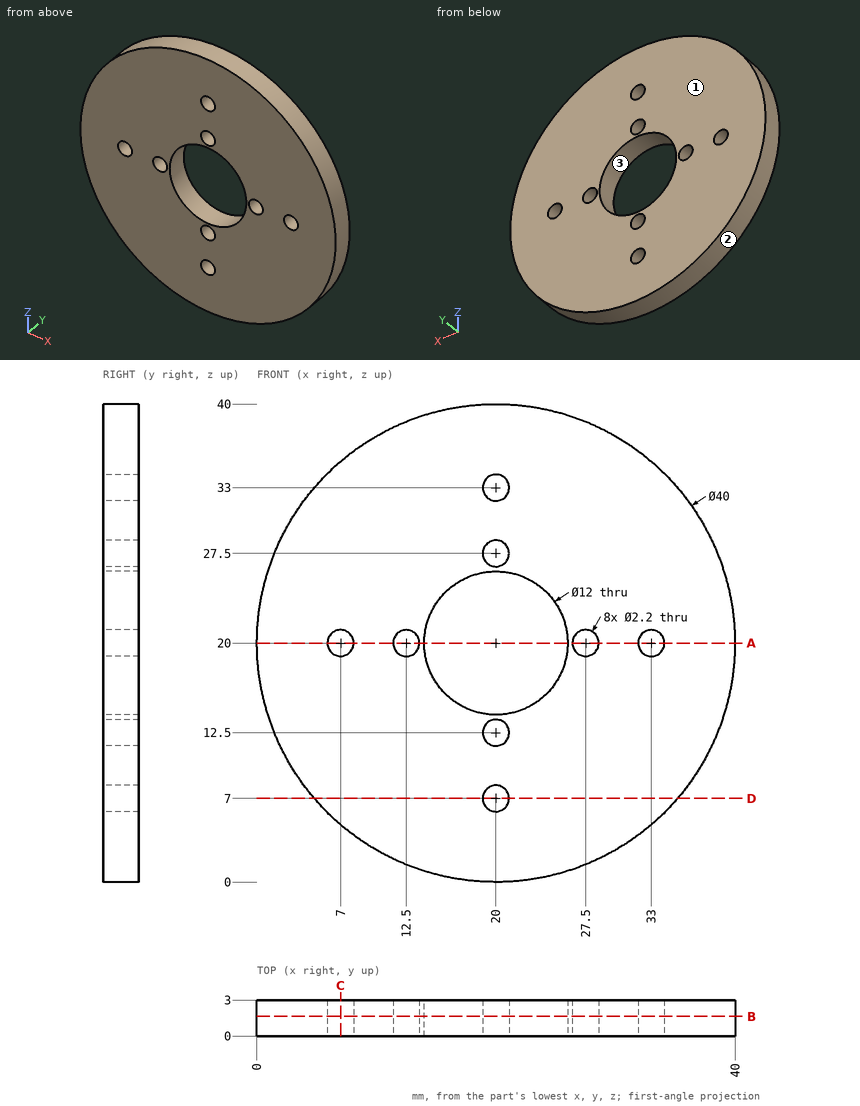
Print and shaded views of the part. All mm, measured from the part's lowest x, y and z. Coordinates: 2 decimals unless noted, no trailing zeros. Order: outer loops, then holes, each group sorted by start corner. A loop starts at its lowest first (then second) coordinate and runs counter-clockwise, first axis right, second up. Notation, with made-up numbers: (0.25, 2) -> (31.25, 2) arc R15 ccw to (31.25, 22) -> close; hole circle Ø5 at (39.25, 6). An arc over 180 degrees is marked (long way). Answer as a JSON object with one key per item and string values. Group by question number.
1) Flat gauge pins, fed straight in: pin 1 (1.5 mm diameter, centred on x = 27, y = 2, fed in from +Z); pin 2 (1.8 mm diameter, centred on x = 20, z = 12.5, fed in from +Y). Where does each tip first touch, or does it go through?
2) Cut at A-A, the plane z = 20. Write the cut outline in (x, y), then the cut area to 3 significant figures.
3) Cut at B-B, the plane y = 1.65. Count the separate pieces of the cut face and the enclosed holes in it, then the cut area to 3 significant figures.
4) Drill centre lines: L1, parallel to Z at x = 20, y = 1.15; L2, parallel to Z at x = 19, y = 2.7; L3, parallel to X at y = 0.3, z = 24.5. Where is each one in solid material? Low to high.
5) Cut at C-C, the plane x = 7. Write the cut outline in (y, z), then the cut area to 3 significant figures.
6) Pull direction X, two halves, no side cores. Call the marked faces 1, 2 and 3: +X half, -X half, draft (parallel to the pull), parting line (faces both ways), or undercut.
7) Cut at D-D, the plane z = 7. Write the cut outline in (x, y), then the cut area to 3 significant figures.
Check values:
{
 "1": {"pin 1": "stops at z = 39", "pin 2": "passes through"},
 "2": {"outline": "(0, 0) -> (5.9, 0) -> (5.9, 3) -> (0, 3) -> close; (8.1, 0) -> (11.4, 0) -> (11.4, 3) -> (8.1, 3) -> close; (13.6, 0) -> (14, 0) -> (14, 3) -> (13.6, 3) -> close; (26, 0) -> (26.4, 0) -> (26.4, 3) -> (26, 3) -> close; (28.6, 0) -> (31.9, 0) -> (31.9, 3) -> (28.6, 3) -> close; (34.1, 0) -> (40, 0) -> (40, 3) -> (34.1, 3) -> close", "area": "57.6 mm²"},
 "3": {"separate pieces": "1", "enclosed holes": "9", "area": "1,110 mm²"},
 "4": {"L1": "z = 0 to 5.9, 8.1 to 11.4, 13.6 to 14, 26 to 26.4, 28.6 to 31.9, 34.1 to 40", "L2": "z = 0.03 to 6.54, 7.46 to 12.04, 12.96 to 14.08, 25.92 to 27.04, 27.96 to 32.54, 33.46 to 39.97", "L3": "x = 0.51 to 16.03, 23.97 to 39.49"},
 "5": {"outline": "(0, 4.8) -> (3, 4.8) -> (3, 18.9) -> (0, 18.9) -> close; (0, 21.1) -> (3, 21.1) -> (3, 35.2) -> (0, 35.2) -> close", "area": "84.6 mm²"},
 "6": {"face 1": "draft", "face 2": "parting line", "face 3": "undercut"},
 "7": {"outline": "(4.8, 0) -> (18.9, 0) -> (18.9, 3) -> (4.8, 3) -> close; (21.1, 0) -> (35.2, 0) -> (35.2, 3) -> (21.1, 3) -> close", "area": "84.6 mm²"}
}
